from build123d import *

# Parameters (mm, degrees)
F0_W      = 479.028125
F0_H      = 167.619304
F0_W_2    = 19.84375
F0_H_2    = 38.89375
F0_W_3    = 285.353125
F0_H_3    = 96.440625
F0_W_4    = 76.99375
F0_H_4    = 19.84375
F0_W_5    = 57.94375
F0_H_5    = 39.290625
F1_DEPTH  = 5.953125
F2_R      = 2.38125
F2_R_2    = 0.79375
F3_DEPTH  = 5.954125
F4_W      = 479.028125
F4_H      = 167.619304
F4_W_2    = 466.328125
F4_H_2    = 154.919304
F5_DEPTH  = 9.525
F6_W      = 34.925
F6_H      = 14.2875
F7_DEPTH  = 15.479125
F9_R      = 0.79375
F10_DEPTH = 42.530125


with BuildPart() as f1:
    # F0 (on Top) → F1 (new body)
    with BuildSketch(Plane.XY):
        with Locations((236.339062, 74.284652)):
            Rectangle(F0_W, F0_H)
        with Locations((16.271875, 25.796875)):
            Rectangle(F0_W_2, F0_H_2, mode=Mode.SUBTRACT)
        with Locations((16.271875, 68.659375)):
            Rectangle(F0_W_2, F0_H_2, mode=Mode.SUBTRACT)
        with Locations((180.776563, 54.570312)):
            Rectangle(F0_W_3, F0_H_3, mode=Mode.SUBTRACT)
        Polygon((385.365625, 6.35), (327.421875, 6.35), (327.421875, 26.19375), (346.471875, 26.19375), (346.471875, 45.640625), (366.315625, 45.640625), (366.315625, 26.19375), (385.365625, 26.19375), align=None, mode=Mode.SUBTRACT)
        with Locations((427.83125, 54.570312)):
            Rectangle(F0_W_4, F0_H_3, mode=Mode.SUBTRACT)
        with Locations((16.271875, 111.521875)):
            Rectangle(F0_W_2, F0_H_2, mode=Mode.SUBTRACT)
        with Locations((48.021875, 121.046875)):
            Rectangle(F0_W_2, F0_H_4, mode=Mode.SUBTRACT)
        with Locations((107.95, 121.046875)):
            Rectangle(F0_W_4, F0_H_4, mode=Mode.SUBTRACT)
        with Locations((196.453125, 121.046875)):
            Rectangle(F0_W_4, F0_H_4, mode=Mode.SUBTRACT)
        with Locations((356.39375, 83.145312)):
            Rectangle(F0_W_5, F0_H_5, mode=Mode.SUBTRACT)
        with Locations((284.95625, 121.046875)):
            Rectangle(F0_W_4, F0_H_4, mode=Mode.SUBTRACT)
        with Locations((356.39375, 121.046875)):
            Rectangle(F0_W_5, F0_H_4, mode=Mode.SUBTRACT)
    extrude(amount=F1_DEPTH)

    # F2 (on face) → F3 (cut, through all)
    with BuildSketch(Plane.XY.offset(5.953125)):
        with Locations((83.34375, 144.859375)):
            Circle(F2_R)
        with Locations((102.39375, 144.859375)):
            Circle(F2_R)
        with Locations((121.44375, 144.859375)):
            Circle(F2_R)
        with Locations((140.49375, 144.859375)):
            Circle(F2_R)
        with Locations((168.275, 144.859375)):
            Circle(F2_R)
        with Locations((294.48125, 144.859375)):
            Circle(F2_R)
        with Locations((309.165625, 144.859375)):
            Circle(F2_R)
        with Locations((332.58125, 144.859375)):
            Circle(F2_R)
        with Locations((351.63125, 144.859375)):
            Circle(F2_R)
        with Locations((370.68125, 144.859375)):
            Circle(F2_R)
        with Locations((389.73125, 144.859375)):
            Circle(F2_R)
        with Locations((405.60625, 116.284375)):
            Circle(F2_R)
        with Locations((405.60625, 132.55625)):
            Circle(F2_R_2)
        with Locations((421.48125, 132.55625)):
            Circle(F2_R_2)
        with Locations((437.35625, 132.55625)):
            Circle(F2_R_2)
        with Locations((453.23125, 132.55625)):
            Circle(F2_R_2)
    extrude(amount=-F3_DEPTH, mode=Mode.SUBTRACT)

    # F4 (on face) → F5 (join)
    with BuildSketch(Plane(origin=(0, 0, 0), x_dir=(1, 0, 0), z_dir=(0, 0, -1))):
        with Locations((236.339062, -74.284652)):
            Rectangle(F4_W, F4_H)
        with Locations((236.339062, -74.284652)):
            Rectangle(F4_W_2, F4_H_2, mode=Mode.SUBTRACT)
    extrude(amount=F5_DEPTH)

    # F6 (on face) → F7 (cut, through all)
    with BuildSketch(Plane.XY.offset(5.953125)):
        with Locations((439.340625, 118.26875)):
            Rectangle(F6_W, F6_H)
    extrude(amount=-F7_DEPTH, mode=Mode.SUBTRACT)

    # F9 (on offset) → F10 (cut, through all)
    with BuildSketch(Plane.YZ.offset(433.324)):
        with Locations((118.26875, -4.7625)):
            Circle(F9_R)
    extrude(amount=F10_DEPTH, mode=Mode.SUBTRACT)


solid = f1.part
Design review of the part built by this model. Coordinates are the model's own, in mm. A direction names the side the tool comes from. Coordinates: 2 decimals unless noted, no trailing zeros. Order: outer loops, then holes, each group sorted by start corner. A loop starts at its lowest first (then second) coordinate and runs counter-clockwise, first axis right, second up. Notation, with made-up numbers: (11.25, -32) -> (35.25, -32) arc R25 cw to (35.25, -13) -> close; hole circle Ø5 at (-36.5, 37.25). An arc over 180 degrees is marked (long way). Use one line per item in the form item = value. Start each with the question number.
(1) For probe 1 along Y at (x, z) = (249, 4.5) (3 decimals); probe 2 along X at (y, z) = (15.5, -5.25) (3 decimals); probe 3 along Y at (x, z) = (311, -7) (3 decimals), list the stretches that pass through material, from the lowest coordinate up.
(2) Add section C-C on x = 431. Give the number of separate pieces and of enclosed holes in the cut face, plus the area to 3 significant figures.
(3) For faces 1 (the flat face through (233, -9.525, -2)), 2 (the flat face through (469.503, 75, -5)), list the 3-axis set-ups (+Z, -Z, +X, -X, +Y, -Y) from which the entire face can be reached by the end or side of a thin tool; tool diameter is ignored.
(4) The part is to be moulded in two halves that separate along Y. For faces 3 (the flat face through (218, 109, 0)), 4 (the flat face through (233, 158.094, -2)), 5 (the flat face through (3.175, 75, -5)), 6 (the flat face through (475.853, 75, -2)), say which applies: +Y half, -Y half, draft (parallel to the pull), parting line (faces both ways), or undercut.
(5) Add section A-A on y = 58. State the section outline as (x, z) points (3 decimals), plus the area to 3 significant figures.
(6) Add section B-B on x = 342. State the section outline as (y, z) points (3 decimals).
(7) Add section D-D on x = 114. State the section outline as (y, z) points (3 decimals), plus the area to 3 significant figures.
Answer block:
q1.probe_1 = -9.525 to 6.35, 102.791 to 111.125, 130.969 to 158.094
q1.probe_2 = -3.175 to 3.175, 469.503 to 475.853
q1.probe_3 = -9.525 to -3.175, 151.744 to 158.094
q2.separate_pieces = 3
q2.enclosed_holes = 0
q2.area = 460 mm²
q3.face_1 = +Z, -Z, +X, -X, -Y
q3.face_2 = -Z
q4.face_3 = undercut
q4.face_4 = +Y half
q4.face_5 = undercut
q4.face_6 = draft
q5.outline = (-3.175, -9.525) -> (3.175, -9.525) -> (3.175, 0) -> (6.35, 0) -> (6.35, 5.953) -> (-3.175, 5.953) -> close; (26.194, 0) -> (38.1, 0) -> (38.1, 5.953) -> (26.194, 5.953) -> close; (323.453, 0) -> (389.334, 0) -> (389.334, 5.953) -> (323.453, 5.953) -> close; (466.328, 0) -> (469.503, 0) -> (469.503, -9.525) -> (475.853, -9.525) -> (475.853, 5.953) -> (466.328, 5.953) -> close
q5.area = 697 mm²
q6.outline = (-9.525, -9.525) -> (-3.175, -9.525) -> (-3.175, 0) -> (6.35, 0) -> (6.35, 5.953) -> (-9.525, 5.953) -> close; (26.194, 0) -> (63.5, 0) -> (63.5, 5.953) -> (26.194, 5.953) -> close; (102.791, 0) -> (111.125, 0) -> (111.125, 5.953) -> (102.791, 5.953) -> close; (130.969, 0) -> (151.744, 0) -> (151.744, -9.525) -> (158.094, -9.525) -> (158.094, 5.953) -> (130.969, 5.953) -> close
q7.outline = (-9.525, -9.525) -> (-3.175, -9.525) -> (-3.175, 0) -> (6.35, 0) -> (6.35, 5.953) -> (-9.525, 5.953) -> close; (102.791, 0) -> (111.125, 0) -> (111.125, 5.953) -> (102.791, 5.953) -> close; (130.969, 0) -> (151.744, 0) -> (151.744, -9.525) -> (158.094, -9.525) -> (158.094, 5.953) -> (130.969, 5.953) -> close
q7.area = 427 mm²
